Work out the finished part from the listing and answer in its coordinate system (mm). A direction names the side the tool comes from. Coordinates: 2 decimals unless noted, no trailing zeros. Order: outer loops, then holes, each group sorted by start corner. A loop starts at its lowest first (then second) coordinate and runs counter-clockwise, first axis right, second up.
1. Find the intervals of material crossed by probe 1 along Z at (x, y) = (23.25, -4); probe 2 along Z at (x, y) = (5, -5.25); probe 3 along Y at (x, z) = (11.25, 7), in increasing order.
2. The part is cut by section A-A, the plane z = 3.75. Give the vertices of the cut face in (x, y) (1 decimal).
3. A tool of negligible diameter and unlimited length cuts with its end or side. For faces 1 (the cylindrical face through (3.43, -8.68, 3.52)), 2 (the flat face through (19, 0, 13)), from which of +Z, -Z, +X, -X, +Y, -Y can it reach the whole face along a straight path? Write none if from no direction.
4. The part is cut by section B-B, the plane z = 7.5. Give the vertices of the cut face in (x, y) (1 decimal).
5. Flat-ended cylindrical pins translate along their axes: pin 1 Ø5 at (y, z) = (-3, 22) entering from -X; pin 2 Ø1 at (y, z) = (8.5, 18.5) entering from +X; pin 3 Ø9 at (x, z) = (21, 12.5) entering from +Y. Find the tip coordinate at first contact, or state that the pin passes through.
```python
from build123d import *

# Parameters (mm, degrees)
F3_DEPTH = 25.401


with BuildPart() as f1:
    # F0 (on Front) → F1 (revolve)
    with BuildSketch(Plane.XZ):
        with BuildLine():
            Line((0, 7.14375), (0, 0))
            Line((0, 0), (12.7, 0))
            Line((12.7, 0), (12.7, 25.4))
            Line((12.7, 25.4), (0, 25.4))
            Line((0, 25.4), (0, 18.25625))
            ThreePointArc((0, 18.25625), (3.928862053, 16.628862053), (5.55625, 12.7))
            ThreePointArc((5.55625, 12.7), (3.928862053, 8.771137947), (0, 7.14375))
        make_face()
    revolve(axis=Axis((12.7, 0, 12.7), (0, 0, 1)))

    # F2 (on face) → F3 (cut, through all)
    with BuildSketch(Plane.XY.offset(25.4)):
        with BuildLine():
            Line((12.7, 1.5875), (12.7, 0))
            Line((12.7, 0), (14.2875, 0))
            ThreePointArc((14.2875, 0), (13.8225320151, 1.1225320151), (12.7, 1.5875))
        make_face()
        with BuildLine():
            Line((14.2875, 0), (12.7, 0))
            Line((12.7, 0), (11.1125, 0))
            ThreePointArc((11.1125, 0), (12.7, -1.5875), (14.2875, 0))
        make_face()
        with BuildLine():
            Line((11.1125, 0), (12.7, 0))
            Line((12.7, 0), (12.7, 1.5875))
            ThreePointArc((12.7, 1.5875), (11.5774679849, 1.1225320151), (11.1125, 0))
        make_face()
        with BuildLine():
            ThreePointArc((12.7, 1.5875), (13.8225320151, 1.1225320151), (14.2875, 0))
            Line((14.2875, 0), (25.4, 0))
            ThreePointArc((25.4, 0), (21.6802561211, 8.9802561211), (12.7, 12.7))
            Line((12.7, 12.7), (12.7, 1.5875))
        make_face()
    extrude(amount=-F3_DEPTH, mode=Mode.SUBTRACT)


solid = f1.part
```
Geometry says:
1. probe 1: z = 0 to 7.33, 18.07 to 25.4
1. probe 2: z = 0 to 8.29, 17.11 to 25.4
1. probe 3: y = -12.62 to -0.65, 0.65 to 12.62
2. outline: (12.7, 1.6) - (12.7, 12.7) arc R12.7 ccw (long way) to (25.4, 0) - (14.3, 0) arc R1.6 cw (long way) to start
3. face 1: +Z, -Z
3. face 2: +Z, -Z, +X, +Y
4. outline: (12.7, 1.6) - (12.7, 10.7) arc R10.7 ccw (long way) to (23.4, 0) - (14.3, 0) arc R1.6 cw (long way) to start
5. pin 1: stops at x = 0.01
5. pin 2: stops at x = 12.7
5. pin 3: stops at y = 0
